Check sheet for the modelled part. Datum: model origin and axes. Units: mm. A direction names the side the tool comes from. Round coordinates to 2 decimals unless told otherwise and drop trailing zeros. Loops run counter-clockwise (first coordinate to the right, second up) from the corner with the lowest first, then second, coordinate; pieces in that order, holes last. Notation, with made-up numbers: (82, 76.25) - (123, 76.25) arc R19 cw to (123, 96.25) - close; hole circle Ø10 at (-1.5, -12). An arc over 180 degrees is marked (long way). Put each result on its own line as item: value.
```python
from build123d import *

# Parameters (mm, degrees)
FASE1_SIZE = 0.5
FASE2_SIZE = 0.2


with BuildPart() as part:
    # Skizze1 → Rotation1 (revolve)
    with BuildSketch(Plane.XY):
        Polygon((0, 0), (0, 3.25), (3, 3.25), (3, 2), (13, 2), (13, 1.25), (18, 1.25), (18, 0), align=None)
    revolve(axis=Axis((0, 0, 0), (1, 0, 0)))

    # Fase1
    fase1_edges = [part.edges().sort_by_distance(p)[0] for p in [
        (0, -3.25, 0),
    ]]
    chamfer(fase1_edges, length=FASE1_SIZE)

    # Fase2
    fase2_edges = [part.edges().sort_by_distance(p)[0] for p in [
        (18, -1.25, 0),
    ]]
    chamfer(fase2_edges, length=FASE2_SIZE)

    # Skizze2 → Schnitt-Rotation1 (revolve, cut)
    with BuildSketch(Plane.XY):
        Polygon((13, 1.25), (13, 1), (13.5, 1), (13.933012702, 1.25), align=None)
    revolve(axis=Axis((0, 0, 0), (1, 0, 0)), mode=Mode.SUBTRACT)


solid = part.part
```
Item 1: Go/stop test with flat-tipped pins: pin 1 (1 mm diameter, centred on x = 6, z = -0.5, fed in from +Y); pin 2 (3 mm diameter, centred on x = 7.5, y = 2.5, fed in from -Z). Record where each tip stops, or that it passes through.
Filled sheet:
pin 1: y = 2
pin 2: z = -1.73
Item 2: Thickness scan on line 1 (X direction, y = -2.25, z = 1.25); line 2 (X direction, y = 0, z = -1.75); line 3 (X direction, y = -0.5, z = 1). Record the ranges inside material, lowest first. Write a range as from..to.
Filled sheet:
line 1: 0..3
line 2: 0..13
line 3: 0..13, 13.7..17.93
Item 3: Section check C-C on x = 6. Enter the section's corners in (y, z).
Filled sheet:
outline: circle Ø4 at (0, 0)
Item 4: Tool access check on faces 4 (the cylindrical face through (1.768, -2.579, -1.978)), 5 (the cylindrical face through (15.89, -0.27, -1.22)). Record the directions out of +Z, -Z, +X, -X, +Y, -Y that give a thin tool (end or side, any length) a straight path to the whole face; none if there is none.
Filled sheet:
face 4: +X, -X
face 5: +X
Item 5: Release check for a two-part mould opening along X. For faces 1 (the cylindrical face through (13.254, -0.217, -0.976)), 2 (the flat face through (18, 0, 0)), 3 (the cylindrical face through (8, 0, -2)) record: +X half, -X half, draft (parallel to the pull), parting line (faces both ways), or undercut.
Filled sheet:
face 1: undercut
face 2: +X half
face 3: draft
Item 6: Section check A-A on y = 0. Enter the section's corners in (x, z), then the cut area to 3 significant figures.
Filled sheet:
outline: (0, -2.75) - (0.5, -3.25) - (3, -3.25) - (3, -2) - (13, -2) - (13, -1) - (13.5, -1) - (13.93, -1.25) - (17.8, -1.25) - (18, -1.05) - (18, 1.05) - (17.8, 1.25) - (13.93, 1.25) - (13.5, 1) - (13, 1) - (13, 2) - (3, 2) - (3, 3.25) - (0.5, 3.25) - (0, 2.75) - close
area: 71.4 mm²
